```python
from build123d import *

# Parameters (mm, degrees)
SKETCH1_R           = 29
SKETCH1_R_2         = 2
BOSS_EXTRUDE1_DEPTH = 5


with BuildPart() as part:
    # Sketch1 → Boss-Extrude1 (new body)
    with BuildSketch(Plane(origin=(0, 0, 0), x_dir=(1, 0, 0), z_dir=(0, 1, 0))):
        with BuildLine():
            Line((-15, 125), (-40.079636882, 8.638443574))
            ThreePointArc((-40.079636882, 8.638443574), (0, -41), (40.079636882, 8.638443574))
            Line((40.079636882, 8.638443574), (15, 125))
            ThreePointArc((15, 125), (0, 140), (-15, 125))
        make_face()
        with Locations(Location((0, 0, 0), (0, 0, 270))):
            Circle(SKETCH1_R, mode=Mode.SUBTRACT)
        with Locations(Location((36, 0, 0), (0, 0, 270))):
            Circle(SKETCH1_R_2, mode=Mode.SUBTRACT)
        with Locations(Location((18, -31.176914536, 0), (0, 0, 270))):
            Circle(SKETCH1_R_2, mode=Mode.SUBTRACT)
        with Locations(Location((-18, -31.176914536, 0), (0, 0, 270))):
            Circle(SKETCH1_R_2, mode=Mode.SUBTRACT)
        with Locations(Location((-36, 0, 0), (0, 0, 270))):
            Circle(SKETCH1_R_2, mode=Mode.SUBTRACT)
        with Locations(Location((-18, 31.176914536, 0), (0, 0, 270))):
            Circle(SKETCH1_R_2, mode=Mode.SUBTRACT)
        with Locations(Location((18, 31.176914536, 0), (0, 0, 270))):
            Circle(SKETCH1_R_2, mode=Mode.SUBTRACT)
    extrude(amount=BOSS_EXTRUDE1_DEPTH)


solid = part.part
```
Verification items for the finished model (mm, model axes). Give positions to 0.01 mm unless a question says otherwise; leave off trailing zeros. Order: outer loops, then holes, each group sorted by start corner. A loop starts at its lowest first (then second) coordinate and runs counter-clockwise, first axis right, second up. Notation, with made-up numbers: (24, -12.5) -> (34, -12.5) arc R19 cw to (34, 3.5) -> close; hole circle Ø8 at (-26.5, 35.25). An arc over 180 degrees is marked (long way). One line per item, written item: value.
(1) Sectioned sample at A-A on x = 0. Record the cut outline in (y, z), then the cut area to 3 significant figures.
Final values:
outline: (0, -140) -> (5, -140) -> (5, -29) -> (0, -29) -> close; (0, 29) -> (5, 29) -> (5, 41) -> (0, 41) -> close
area: 615 mm^2
(2) Scan lines: line 1 along X through (y, z) = (2.65, 0); line 2 along X through (y, z) = (3.95, 22); line 3 along X through (y, z) = (4.45, -125). Record each from-to range of solid material in increasing order. Write a range as [from, to].
Final values:
line 1: [-41, -38], [-34, -29], [29, 34], [38, 41]
line 2: [-34.6, -18.89], [18.89, 34.6]
line 3: [-15, 15]
(3) Gauge pin test, flat ends, axial feed: pin 1 (5 mm diameter, centred on x = 18, z = -31.18, fed in from +Y); pin 2 (1 mm diameter, centred on y = 3, z = -42, fed in from -X); pin 3 (1 mm diameter, centred on x = 19.5, y = 1, fed in from +Z). Record the tip position at first contact, or that the pin passes through.
Final values:
pin 1: y = 5
pin 2: x = -33
pin 3: z = 36.33
(4) Sectioned sample at C-C on x = 18. Record the cut outline in (y, z), then the cut area to 3 significant figures.
Final values:
outline: (0, -111.08) -> (5, -111.08) -> (5, -33.18) -> (0, -33.18) -> close; (0, -29.18) -> (5, -29.18) -> (5, -22.74) -> (0, -22.74) -> close; (0, 22.74) -> (5, 22.74) -> (5, 29.18) -> (0, 29.18) -> close; (0, 33.18) -> (5, 33.18) -> (5, 36.84) -> (0, 36.84) -> close
area: 472 mm^2
(5) Draft check along X on faces 1 (the face through (-1, 0, -51)), 2 (the face through (-16.017, 2.465, 30.917)), 3 (the face through (-1.023, 2.465, 40.987)). Enter one of: pulls with the +X half, pulls with the -X half, needs draft (parallel to the pull), parting line crosses it, or undercut.
Final values:
face 1: needs draft
face 2: undercut
face 3: parting line crosses it
(6) Sectioned sample at B-B on z = 0. Record the cut outline in (x, y), then the cut area to 3 significant figures.
Final values:
outline: (-41, 0) -> (-38, 0) -> (-38, 5) -> (-41, 5) -> close; (-34, 0) -> (-29, 0) -> (-29, 5) -> (-34, 5) -> close; (29, 0) -> (34, 0) -> (34, 5) -> (29, 5) -> close; (38, 0) -> (41, 0) -> (41, 5) -> (38, 5) -> close
area: 80.0 mm^2
(7) Sectioned sample at D-D on z = -20. Record the cut outline in (x, y), then the cut area to 3 significant figures.
Final values:
outline: (-37.63, 0) -> (-21, 0) -> (-21, 5) -> (-37.63, 5) -> close; (21, 0) -> (37.63, 0) -> (37.63, 5) -> (21, 5) -> close
area: 166 mm^2
